Verification items for the finished model (mm, model axes). A direction names the side the tool comes from. Give positions to 0.01 mm unless a question says otherwise; leave off trailing zeros. Loops run counter-clockwise (first coordinate to the right, second up) from the corner with the lowest first, then second, coordinate; pieces in that order, holes last. Notation, with made-up numbers: M 18.5,52.25 L 49.5,52.25 A25 ccw 49.5,64.25 Z; hole C -14.5,6 d1. An arc over 180 degrees is marked long. Use CSV: the item, a comma, the result in double quotes.
from build123d import *

# Parameters (mm, degrees)
SCHIZZO1_R                    = 16
ESTRUSIONE_ESTRUSIONE1_DEPTH  = 20
SMUSSO1_SIZE                  = 3
TAGLIO_ESTRUSIONE1_DEPTH      = 31.199337741
TAGLIO_ESTRUSIONE1_DEPTH_BACK = 31.199337741
SCHIZZO2_R                    = 3
SCHIZZO3_R                    = 9
ESTRUSIONE_ESTRUSIONE2_DEPTH  = 135
SCHIZZO4_W                    = 1.3
SCHIZZO4_H                    = 0.85


with BuildPart() as part:
    # Schizzo1 → Estrusione-Estrusione1 (new body)
    with BuildSketch(Plane.XY):
        Circle(SCHIZZO1_R)
    extrude(amount=ESTRUSIONE_ESTRUSIONE1_DEPTH)

    # Smusso1
    smusso1_edges = [part.edges().sort_by_distance(p)[0] for p in [
        (-16, 0, 0),
        (-16, 0, 20),
    ]]
    chamfer(smusso1_edges, length=SMUSSO1_SIZE)

    # Schizzo2 → Taglio-Estrusione1 (cut, two sides: drawn at the far end of the back side and taken through both)
    with BuildSketch(Plane(origin=(0, 0, 0), x_dir=(0, 0, -1), z_dir=(1, 0, 0)).offset(-TAGLIO_ESTRUSIONE1_DEPTH_BACK)):
        with Locations((-10, 0)):
            Circle(SCHIZZO2_R)
    extrude(amount=TAGLIO_ESTRUSIONE1_DEPTH + TAGLIO_ESTRUSIONE1_DEPTH_BACK, mode=Mode.SUBTRACT)

    # Schizzo3 → Estrusione-Estrusione2 (add)
    with BuildSketch(Plane.XY):
        Circle(SCHIZZO3_R)
    extrude(amount=-ESTRUSIONE_ESTRUSIONE2_DEPTH)

    # Schizzo4 → Taglia-Rivoluzione1 (revolve, cut)
    with BuildSketch(Plane(origin=(0, 0, 0), x_dir=(0, 0, -1), z_dir=(1, 0, 0)), mode=Mode.PRIVATE) as taglia_rivoluzione1_sk:
        with Locations((52.15, 8.575)):
            Rectangle(SCHIZZO4_W, SCHIZZO4_H)
        with Locations((73.25, 8.575)):
            Rectangle(SCHIZZO4_W, SCHIZZO4_H)
    revolve(taglia_rivoluzione1_sk.sketch.rotate(Axis((0, 0, 0), (0, 0, -1)), 90), axis=Axis((0, 0, 0), (0, 0, -1)), mode=Mode.SUBTRACT)


solid = part.part
(1) Scan lines: L1, parallel to Z at x = -7, y = 0; L2, parallel to Z at x = -8.5, y = 2; L3, parallel to Z at x = 5, y = -1.5. Record each from-to range of solid material in increasing order. Write a range as from..to.
Calculated:
L1,"z = -135..7, 13..20"
L2,"z = -135..-73.9, -72.6..-52.8, -51.5..7.76, 12.24..20"
L3,"z = -135..7.4, 12.6..20"
(2) Mould release check, pull along Z, two halves, no side actions. Record for faces 4 (the cylindrical face through (-0.2, -1.8, 12.4)), 5 (the cylindrical face through (-1.172, 8.923, -104.022)), 6 (the flat face through (3, 9, 0)): released by +Z, released by -Z, zero draft, split by the parting line, or undercut.
Calculated:
face 4,"undercut"
face 5,"zero draft"
face 6,"released by -Z"
(3) Section check C-C on z = 10. Record the cut outline in (x, y), plus the area to 3 significant figures.
Calculated:
outline,"M -15.72,-3 A16 ccw 15.72,-3 Z; M -15.72,3 L 15.72,3 A16 ccw Z"
area,"613 mm²"
(4) Tool access check on faces 1 (the flat face through (5, -7, -72.6)), 2 (the cylindrical face through (-1.172, 8.923, -25.39)), 3 (the flat face through (0, 0, 20)). Record the directions out of +Z, -Z, +X, -X, +Y, -Y that give a thin tool (end or side, any length) a straight path to the whole face; none if there is none.
Calculated:
face 1,"none"
face 2,"-Z"
face 3,"+Z, +X, -X, +Y, -Y"
(5) Section check D-D on z = -6. Record the cut outline in (x, y), plus the area to 3 significant figures.
Calculated:
outline,"C 0,0 d18"
area,"254 mm²"
(6) Depth check by flat-ended pin: pin 1 Ø10 at (y, z) = (1.5, -113.5) entering from +X; pin 2 Ø8 at (y, z) = (0, 10) entering from +X; pin 3 Ø3 at (y, z) = (8, -50.5) entering from +X; pin 4 Ø8 at (x, z) = (10, -47) entering from +Y. Enter the tip coordinate at first touch or a pass-through.
Calculated:
pin 1,"stops at x = 9"
pin 2,"stops at x = 16"
pin 3,"stops at x = 6.22"
pin 4,"stops at y = 6.71"
